from build123d import *

# Parameters (mm, degrees)
SKETCH1_R           = 127
BOSS_EXTRUDE1_DEPTH = 6.35
SKETCH2_R           = 50.8
CUT_EXTRUDE1_DEPTH  = 6.35
SKETCH4_R           = 12.7
CUT_EXTRUDE4_DEPTH  = 12.7


with BuildPart() as part:
    # Sketch1 → Boss-Extrude1 (new body)
    with BuildSketch(Plane(origin=(0, 0, 0), x_dir=(1, 0, 0), z_dir=(0, 1, 0))):
        with Locations(Location((0, 0, 0), (0, 0, 270))):
            Circle(SKETCH1_R)
    extrude(amount=BOSS_EXTRUDE1_DEPTH)

    # Sketch2 → Cut-Extrude1 (cut)
    with BuildSketch(Plane(origin=(0, 6.35, 0), x_dir=(1, 0, 0), z_dir=(0, 1, 0))):
        with Locations(Location((0, 0, 0), (0, 0, 270))):
            Circle(SKETCH2_R)
    extrude(amount=-CUT_EXTRUDE1_DEPTH, mode=Mode.SUBTRACT)

    # Sketch4 → Cut-Extrude4 (cut)
    with BuildSketch(Plane(origin=(0, 6.35, 0), x_dir=(1, 0, 0), z_dir=(0, 1, 0))):
        with Locations(Location((0, 107.95, 0), (0, 0, 270))):
            Circle(SKETCH4_R)
        with Locations(Location((93.6625, 53.975, 0), (0, 0, 270))):
            Circle(SKETCH4_R)
        with Locations(Location((0, -107.95, 0), (0, 0, 270))):
            Circle(SKETCH4_R)
        with Locations(Location((-93.6625, 53.975, 0), (0, 0, 270))):
            Circle(SKETCH4_R)
        with Locations(Location((-93.6625, -53.975, 0), (0, 0, 270))):
            Circle(SKETCH4_R)
        with Locations(Location((93.6625, -53.975, 0), (0, 0, 270))):
            Circle(SKETCH4_R)
    extrude(amount=-CUT_EXTRUDE4_DEPTH, mode=Mode.SUBTRACT)


solid = part.part
Can you work these out from the model? Positions are in its coordinate system, mm. Give positions to 0.01 mm unless a question says otherwise; leave off trailing zeros. Loops run counter-clockwise (first coordinate to the right, second up) from the corner with the lowest first, then second, coordinate; pieces in that order, holes last. Notation, with made-up numbers: (71.25, 47.25) - (115.25, 47.25) arc R27 ccw to (115.25, 84.25) - close; hole circle Ø11 at (-14, 3.5). An arc over 180 degrees is marked (long way). Return JSON: item names as keys, results as strings.
1. I want a section at C-C on x = -85. Please give me the cut outline in (y, z), and give its area (3 significant figures).
Output values:
{"outline": "(0, -94.36) - (6.35, -94.36) - (6.35, -63.26) - (0, -63.26) - close; (0, -44.69) - (6.35, -44.69) - (6.35, 44.69) - (0, 44.69) - close; (0, 63.26) - (6.35, 63.26) - (6.35, 94.36) - (0, 94.36) - close", "area": "962 mm²"}
2. I want a section at B-B on x = 0. Please give me the cut outline in (y, z).
Output values:
{"outline": "(0, -127) - (6.35, -127) - (6.35, -120.65) - (0, -120.65) - close; (0, -95.25) - (6.35, -95.25) - (6.35, -50.8) - (0, -50.8) - close; (0, 50.8) - (6.35, 50.8) - (6.35, 95.25) - (0, 95.25) - close; (0, 120.65) - (6.35, 120.65) - (6.35, 127) - (0, 127) - close"}
3. I'm going to push flat-ended pins straight in: pin 1 Ø3 at (x, y) = (-72.5, 5.5) entering from +Z; pin 2 Ø1.5 at (x, y) = (30, 3.5) entering from -Z; pin 3 Ø3 at (y, z) = (5.5, -88) entering from -X. Where does each tip first touch, or does it pass through?
Output values:
{"pin 1": "stops at z = 105.3", "pin 2": "stops at z = -123.59", "pin 3": "stops at x = -92.99"}
4. If I drill on line 1 (Z direction, x = 93, y = 5.25); line 2 (Z direction, x = 103, y = 4); line 3 (Z direction, x = -5.5, y = 2.5), over which ranges is the centre line in solid material (lowest first)?
Output values:
{"line 1": "z = -86.49 to -66.66, -41.29 to 41.29, 66.66 to 86.49", "line 2": "z = -74.3 to -62.58, -45.37 to 45.37, 62.58 to 74.3", "line 3": "z = -126.88 to -119.4, -96.5 to -50.5, 50.5 to 96.5, 119.4 to 126.88"}
5. We'd pull the mould along Z, two halves only. Please class faces 1 (the face through (-123.98, 3.13, -27.53)), 2 (the face through (-89.85, 3.22, 66.09)), 3 (the face through (-55, 6.35, -2)): +Z half, -Z half, draft (parallel to the pull), parting line (faces both ways), or undercut.
Output values:
{"face 1": "parting line", "face 2": "undercut", "face 3": "draft"}
6. I want a section at D-D on x = 30. Please give me the cut outline in (y, z).
Output values:
{"outline": "(0, -123.41) - (6.35, -123.41) - (6.35, -41) - (0, -41) - close; (0, 41) - (6.35, 41) - (6.35, 123.41) - (0, 123.41) - close"}
7. I want a section at A-A on z = 0. Please give me the cut outline in (x, y), and give its area (3 significant figures).
Output values:
{"outline": "(-127, 0) - (-50.8, 0) - (-50.8, 6.35) - (-127, 6.35) - close; (50.8, 0) - (127, 0) - (127, 6.35) - (50.8, 6.35) - close", "area": "968 mm²"}
